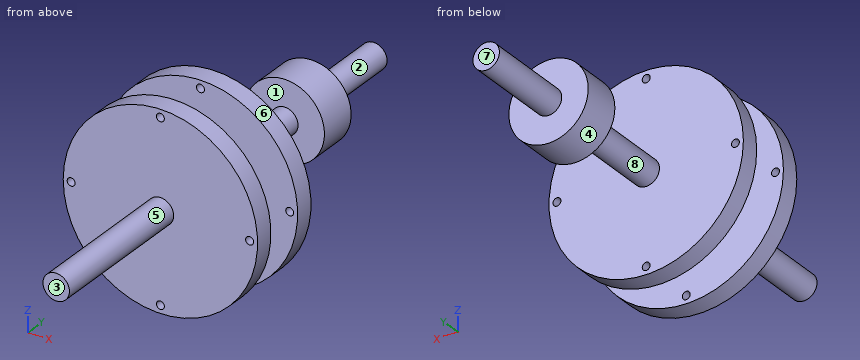
```python
from build123d import *

# Parameters (mm, degrees)
SKETCH1_W          = 10
SKETCH1_H          = 30
SKETCH1_W_2        = 20
SKETCH1_H_2        = 70
SKETCH2_R          = 3
CUT_EXTRUDE1_DEPTH = 80


with BuildPart() as part:
    # Sketch1 → Revolve3 (revolve)
    with BuildSketch(Plane.XY, mode=Mode.PRIVATE) as revolve3_sk:
        Polygon((0, 78.35475), (0, -178.35475), (10, -178.35475), (10, -61.35475), (73.5, -61.35475), (73.5, -46.35475), (10, -46.35475), (10, -16.35475), (73.5, -16.35475), (73.5, -1.35475), (10, -1.35475), (10, 78.35475), align=None)
        with Locations((5, 93.35475)):
            Rectangle(SKETCH1_W, SKETCH1_H)
        with Locations((20, 93.35475)):
            Rectangle(SKETCH1_W_2, SKETCH1_H)
        with Locations((5, 143.35475)):
            Rectangle(SKETCH1_W, SKETCH1_H_2)
    revolve(revolve3_sk.sketch.rotate(Axis((0, 223.956756344, 0), (0, -1, 0)), 180), axis=Axis((0, 223.956756344, 0), (0, -1, 0)))

    # Sketch2 → Cut-Extrude1 (cut)
    with BuildSketch(Plane.XZ.offset(61.35475)):
        with Locations((67.5, 0)):
            Circle(SKETCH2_R)
        with Locations((-67.5, 0)):
            Circle(SKETCH2_R)
        with Locations((0, 67.5)):
            Circle(SKETCH2_R)
        with Locations((0, -67.5)):
            Circle(SKETCH2_R)
    extrude(amount=-CUT_EXTRUDE1_DEPTH, mode=Mode.SUBTRACT)


solid = part.part
```
Input: part model. Units: mm. Frame: model coordinates. Face numbers are marked on the shaded views. A direction names the side the tool comes from. Coordinates: 2 decimals unless noted, no trailing zeros. Loops run counter-clockwise (first coordinate to the right, second up) from the corner with the lowest first, then second, coordinate; pieces in that order, holes last.
Q1. Mould query, pull axis Y, two halves, no side actions, for the marked faces 1, 2 and 3. Classes: +Y half, -Y half, draft (parallel to the pull), parting line (faces both ways), or undercut.
Results are:
face 1: undercut
face 2: draft
face 3: -Y half
Q2. Section D-D, the plane y = -53.5. Return the cut outline in (x, z).
Results are:
outline: circle Ø147 at (0, 0); hole circle Ø6 at (-67.5, 0); hole circle Ø6 at (0, -67.5); hole circle Ø6 at (0, 67.5); hole circle Ø6 at (67.5, 0)
Q3. Line query: line 1 along Z through (x, y) = (0, -10.5); line 2 along Y through (x, z) = (-18, 3.5); line 3 along Y through (x, z) = (-0.5, 31.5). Output: solid intervals per line, ascending.
Results are:
line 1: z = -73.5 to -70.5, -64.5 to 64.5, 70.5 to 73.5
line 2: y = -61.35 to -46.35, -16.35 to -1.35, 78.35 to 108.35
line 3: y = -61.35 to -46.35, -16.35 to -1.35
Q4. Set-up query: the marked faces 4, 5, 6, 7 and 8. Return all of +Z, -Z, +X, -X, +Y, -Y with unobstructed straight access to the full face (end or side cutting, diameter ignored); none if empty.
Results are:
face 4: +Y
face 5: -Y
face 6: +Y, -Y
face 7: +Z, -Z, +X, -X, +Y
face 8: none
Q5. Section A-A, the plane x = 23. Return the cut outline in (y, z), and give its area (3 significant figures).
Results are:
outline: (-61.35, -69.81) - (-46.35, -69.81) - (-46.35, 69.81) - (-61.35, 69.81) - close; (-16.35, -69.81) - (-1.35, -69.81) - (-1.35, 69.81) - (-16.35, 69.81) - close; (78.35, -19.26) - (108.35, -19.26) - (108.35, 19.26) - (78.35, 19.26) - close
area: 5,340 mm2
Q6. Section C-C, the plane z = 24.5. Return the cut outline in (x, y), and give its area (3 significant figures).
Results are:
outline: (-69.3, -61.35) - (69.3, -61.35) - (69.3, -46.35) - (-69.3, -46.35) - close; (-69.3, -16.35) - (69.3, -16.35) - (69.3, -1.35) - (-69.3, -1.35) - close; (-17.31, 78.35) - (17.31, 78.35) - (17.31, 108.35) - (-17.31, 108.35) - close
area: 5,200 mm2
Q7. Section B-B, the plane x = -58. Return the cut outline in (y, z), and give its area (3 significant figures).
Results are:
outline: (-61.35, -45.15) - (-46.35, -45.15) - (-46.35, 45.15) - (-61.35, 45.15) - close; (-16.35, -45.15) - (-1.35, -45.15) - (-1.35, 45.15) - (-16.35, 45.15) - close
area: 2,710 mm2
Q8. Contact query for flat-ended pins moving along their axis: pin 1 (5 mm diameter, centred on x = 67.5, z = 0, fed in from +Y); pin 2 (1.5 mm diameter, centred on y = 40.5, z = -0.5, fed in from -X); pin 3 (1 mm diameter, centred on y = 97, z = 15, fed in from -X); pin 4 (9.5 mm diameter, centred on x = -67.5, z = 0, fed in from -Y). Output: stop coordinate, or through.
Results are:
pin 1: passes through
pin 2: stops at x = -10
pin 3: stops at x = -26.26
pin 4: stops at y = -61.35
